Check sheet for the modelled part. Datum: model origin and axes. Units: mm. Face numbers are marked on the shaded views. Round coordinates to 2 decimals unless told otherwise and drop trailing zeros. Write each loop counter-clockwise with the first axis right and the second up, starting at its lowest first coordinate (ties: lowest second). Pieces come first, ordered by that corner, then holes. Notation, with made-up numbers: (24, 36) - (42, 36) arc R25 cw to (42, 55) - close; hole circle Ø4 at (42.25, -14). An arc over 180 degrees is marked (long way). Answer as a JSON object with one key per item and string values. Group by question number.
Item 1: Thickness scan on line 1 (Y direction, x = 0, z = 4); line 2 (X direction, y = -0.1, z = 1); line 3 (X direction, y = 0.6, z = 1). Record the ranges inside material, lowest first.
Item 2: Gauge pin test, flat end, axial feed: P1, Ø1.5, axis at y = -0.5, z = 1.5, coming from the +X side. Record the tip position at first contact, or that the pin passes through.
Item 3: Sectioned sample at B-B on z = 0.5. Record the boundary of the cut face in (x, y).
Item 4: Sectioned sample at C-C on y = -0.4. Record the boundary of the cut face in (x, z).
Item 5: Release check for a two-part mould opening along Y. For the marked faces 1, 2 and 3 record: pulls with the +Y half, pulls with the -Y half, needs draft (parallel to the pull), parting line crosses it, or undercut.
Item 6: Sectioned sample at D-D on y = 1.4. Record the boundary of the cut face in (x, z).
Item 7: Sectioned sample at A-A on x = 0. Record the boundary of the cut face in (y, z), plus the area to 3 significant figures.
Autodesk Inventor part; units mm, degrees
ref_plane "YZ Plane" through (0, 0, 0) normal (1, 0, 0) x (0, 1, 0)
ref_plane "XZ Plane" through (0, 0, 0) normal (0, 1, 0) x (-1, 0, 0)
ref_plane "XY Plane" through (0, 0, 0) normal (0, 0, 1) x (1, 0, 0)
sketch "Sketch1" plane through (0, 0, 0) normal (0, 0, 1) x (1, 0, 0)
  line L0 (2.7496, 0) -> (1.3748, -2.3812)
  line L1 (1.3748, -2.3812) -> (-1.3748, -2.3812)
  line L2 (-1.3748, -2.3812) -> (-2.7496, 0)
  line L3 (-2.7496, 0) -> (-1.3748, 2.3813)
  line L4 (-1.3748, 2.3813) -> (1.3748, 2.3813)
  line L5 (1.3748, 2.3813) -> (2.7496, 0)
  point P0 (0, 0)
  point P1 (0, 0)
  dimension "Diameter" = 4.7625
extrude "Extrusion1" add sketch "Sketch1" along normal blind 6.35
sketch "Sketch2" plane through (0, 0, 6.35) normal (0, 0, 1) x (1, 0, 0)
  point P0 (0, 0)
  point P1 (0, 0)
hole "Hole1" at (0, 0, 6.35) direction (0, 0, -1) diameter 2.6416 end through all
properties part number "standoffiPart-01"
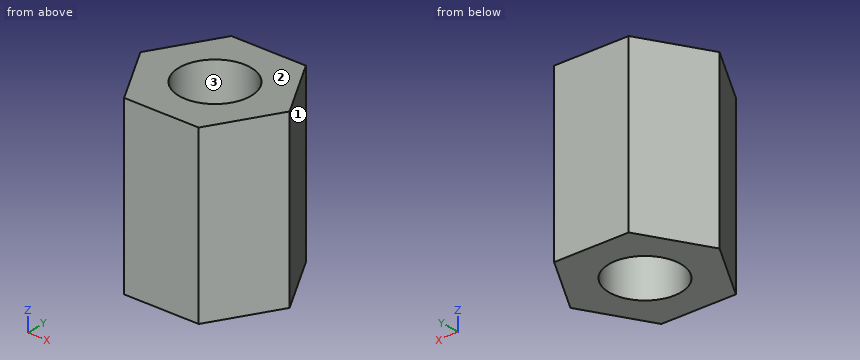
Completed:
{
 "1": {"line 1": "-2.38 to -1.32, 1.32 to 2.38", "line 2": "-2.69 to -1.32, 1.32 to 2.69", "line 3": "-2.4 to -1.18, 1.18 to 2.4"},
 "2": {"P1": "x = 2.75"},
 "3": {"outline": "(-2.75, 0) - (-1.37, -2.38) - (1.37, -2.38) - (2.75, 0) - (1.37, 2.38) - (-1.37, 2.38) - close; hole circle Ø2.64 at (0, 0)"},
 "4": {"outline": "(-2.52, 0) - (-1.26, 0) - (-1.26, 6.35) - (-2.52, 6.35) - close; (1.26, 0) - (2.52, 0) - (2.52, 6.35) - (1.26, 6.35) - close"},
 "5": {"face 1": "pulls with the +Y half", "face 2": "needs draft", "face 3": "undercut"},
 "6": {"outline": "(-1.94, 0) - (1.94, 0) - (1.94, 6.35) - (-1.94, 6.35) - close"},
 "7": {"outline": "(-2.38, 0) - (-1.32, 0) - (-1.32, 6.35) - (-2.38, 6.35) - close; (1.32, 0) - (2.38, 0) - (2.38, 6.35) - (1.32, 6.35) - close", "area": "13.5 mm²"}
}
